```python
from build123d import *

# Parameters (mm, degrees)
F0_W      = 20
F0_H      = 20
F1_DEPTH  = 10
F2_R      = 3.5
F3_DEPTH  = 20.001
F4_R      = 3
F5_DEPTH  = 35
F7_DEPTH  = 4
F11_W     = 65
F11_H     = 56
F12_DEPTH = 52
F13_R     = 1.75
F14_DEPTH = 25


# Not quite as in the source:
# - an extrude whose draft closes it to a point is written as a loft to that point


with BuildPart() as f1:
    # F0 (on Top) → F1 (new body)
    with BuildSketch(Plane.XY):
        Rectangle(F0_W, F0_H)
    extrude(amount=F1_DEPTH)

    # F2 (on face) → F3 (cut, through all)
    with BuildSketch(Plane.YZ.offset(10)):
        with Locations((4, 5)):
            Circle(F2_R)
    extrude(amount=-F3_DEPTH, mode=Mode.SUBTRACT)

    # F4 (on face) → F5 (join)
    with BuildSketch(Plane.XY.offset(10)):
        with Locations((0, -3)):
            Circle(F4_R)
    extrude(amount=F5_DEPTH)

    # F6 (on face) → F7 (join)
    with BuildSketch(Plane(origin=(0, 0, 0), x_dir=(1, 0, 0), z_dir=(0, 0, -1))):
        Polygon((-3.4641016151, 3), (-1.7320508076, 0), (1.7320508076, 0), (3.4641016151, 3), (1.7320508076, 6), (-1.7320508076, 6), align=None)
    extrude(amount=F7_DEPTH)

    # F7_face (on face) → F8 section 0
    with BuildSketch(Plane(origin=(0, -3, -4), x_dir=(1, 0, 0), z_dir=(0, 0, -1)), mode=Mode.PRIVATE) as f8_s0:
        Polygon((-1.7320508076, 3), (-3.4641016151, 0), (-1.7320508076, -3), (1.7320508076, -3), (3.4641016151, 0), (1.7320508076, 3), align=None)
    loft([f8_s0.sketch, Vertex(0, -3, -7)], ruled=True)

    # F11 (on offset) → F12 (join)
    with BuildSketch(Plane.XY.offset(28)):
        with Locations((22.5, -6)):
            Rectangle(F11_W, F11_H)
    extrude(amount=F12_DEPTH)

    # F13 (on face) → F14 (cut)
    with BuildSketch(Plane.XZ.offset(34)):
        with Locations((0, 75)):
            Circle(F13_R)
        with Locations((45, 38)):
            Circle(F13_R)
    extrude(amount=-F14_DEPTH, mode=Mode.SUBTRACT)


solid = f1.part
```
Input: part model. Units: mm. Frame: model coordinates. A direction names the side the tool comes from. Give positions to 0.01 mm unless a question says otherwise; leave off trailing zeros. Order: outer loops, then holes, each group sorted by start corner. A loop starts at its lowest first (then second) coordinate and runs counter-clockwise, first axis right, second up. Notation, with made-up numbers: M -29.5,-31.75 L -6.5,-31.75 A17 ccw -6.5,-11.75 Z; hole C 70.25,-17 d3. An arc over 180 degrees is marked long. Return JSON: item names as keys, results as strings.
1) Access query for faces 1 (the face through (0, -9, 75)), 2 (the face through (2.6, -1.5, -2)), 3 (the face through (0, -10, 5)), 4 (the face through (0, 10, 5)). Directions: +Z, -Z, +X, -X, +Y, -Y. A direction counts if a zero-diameter tool reaches every point of the face in a straight line with its end or side. Return the directions, or none.
Taken from the geometry:
{"face 1": "-Y", "face 2": "-Z, +X, +Y", "face 3": "-Z, +X, -X, -Y", "face 4": "-Z, +X, -X, +Y"}
2) Section query C-C on z = 16. Output: boundary loops of the cut face in (x, y), and give its area (3 significant figures).
Taken from the geometry:
{"outline": "C 0,-3 d6", "area": "28.3 mm2"}
3) Section query D-D on x = 21.5. Output: boundary loops of the cut face in (y, z).
Taken from the geometry:
{"outline": "M -34,28 L 22,28 L 22,80 L -34,80 Z"}
4) Contact query for flat-ended pins moving along their axis: pin 1 (8 mm diameter, centred on y = 2, z = 6, fed in from +X); pin 2 (5 mm diameter, centred on x = 1.5, z = 6.5, fed in from +Y); pin 3 (1.8 mm diameter, centred on x = 0.5, z = 74.5, fed in from -Y); pin 4 (6.5 mm diameter, centred on y = 4, z = 5, fed in from +X). Output: stop coordinate, or through.
Taken from the geometry:
{"pin 1": "stops at x = 10", "pin 2": "stops at y = 10", "pin 3": "stops at y = -9", "pin 4": "passes through"}
5) Line query: L1, parallel to Z at x = 0, y = -17; L2, parallel to Z at x = 0, y = 4; L3, parallel to Z at x = -2.5, y = 9. Output: solid intervals per line, ascending. Write a range as [from, to].
Taken from the geometry:
{"L1": "z = [28, 73.25], [76.75, 80]", "L2": "z = [0, 1.5], [8.5, 10], [28, 80]", "L3": "z = [0, 10], [28, 80]"}
6) Section query B-B on y = -7. Output: boundary loops of the cut face in (x, z), and give its area (3 significant figures).
Taken from the geometry:
{"outline": "M -10,0 L 10,0 L 10,10 L -10,10 Z; M -10,28 L 55,28 L 55,80 L -10,80 Z", "area": "3,580 mm2"}
7) Section query A-A on z = 5. Output: boundary loops of the cut face in (x, y), and give its area (3 significant figures).
Taken from the geometry:
{"outline": "M -10,-10 L 10,-10 L 10,0.5 L -10,0.5 Z; M -10,7.5 L 10,7.5 L 10,10 L -10,10 Z", "area": "260 mm2"}
8) Mould query, pull axis X, two halves, no side actions, for faces 5 (the face through (45, -9, 38)), 6 (the face through (-2.6, -1.5, -2)), 7 (the face through (0, -6, -2)), 8 (the face through (-0.38, -21.68, 73.29)). Classes: released by +X, released by -X, zero draft, split by the parting line, or undercut.
Taken from the geometry:
{"face 5": "undercut", "face 6": "released by -X", "face 7": "zero draft", "face 8": "undercut"}
